```python
from build123d import *

# Parameters (mm, degrees)
SKETCH1_R           = 25
BOSS_EXTRUDE1_DEPTH = 2
SKETCH2_R           = 20
BOSS_EXTRUDE2_DEPTH = 10
SKETCH3_R           = 25
BOSS_EXTRUDE3_DEPTH = 2
SKETCH4_R           = 3.5
CUT_EXTRUDE1_DEPTH  = 19


with BuildPart() as part:
    # Sketch1 → Boss-Extrude1 (new body)
    with BuildSketch(Plane(origin=(0, 0, 0), x_dir=(0, 0, -1), z_dir=(1, 0, 0))):
        Circle(SKETCH1_R)
    extrude(amount=BOSS_EXTRUDE1_DEPTH)

    # Sketch2 → Boss-Extrude2 (add)
    with BuildSketch(Plane(origin=(2, 0, 0), x_dir=(0, 0, -1), z_dir=(1, 0, 0))):
        Circle(SKETCH2_R)
    extrude(amount=BOSS_EXTRUDE2_DEPTH)

    # Sketch3 → Boss-Extrude3 (add)
    with BuildSketch(Plane(origin=(12, 0, 0), x_dir=(0, 0, -1), z_dir=(1, 0, 0))):
        Circle(SKETCH3_R)
    extrude(amount=BOSS_EXTRUDE3_DEPTH)

    # Sketch4 → Cut-Extrude1 (cut)
    with BuildSketch(Plane.ZY):
        Circle(SKETCH4_R)
    extrude(amount=-CUT_EXTRUDE1_DEPTH, mode=Mode.SUBTRACT)


solid = part.part
```
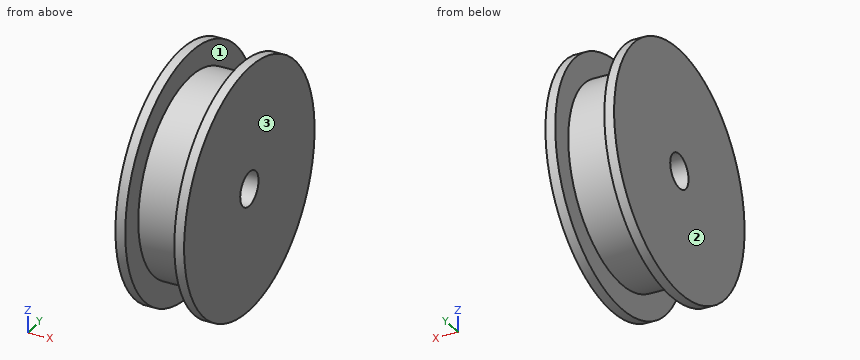
Geometry check sheet. Reference: the model listing, model coordinates, mm. Face numbers are marked on the shaded views. Give positions to 0.01 mm unless a question says otherwise; leave off trailing zeros. Order: outer loops, then holes, each group sorted by start corner. A loop starts at its lowest first (then second) coordinate and runs counter-clockwise, first axis right, second up.
1. Release check for a two-part mould opening along X. For the marked faces 1, 2 and 3 record: pulls with the +X half, pulls with the -X half, needs draft (parallel to the pull), parting line crosses it, or undercut.
2. Section check C-C, the plane x = 4.75. Enter the section's corners in (y, z).
3. Section check A-A, the plane z = 0. Enter the section's corners in (x, y).
4. Thickness scan on L1, parallel to Y at x = 7.75, z = 0; L2, parallel to X at y = 18.5, z = 10.5; L3, parallel to Z at x = 11.5, y = -14. Record the ranges inside material, lowest first.
5. Section check D-D, the plane z = 22.5. Enter the section's corners in (x, y), and give its area (3 significant figures).
6. Gauge pin test, flat ends, axial feed: pin 1 Ø3 at (x, y) = (3, -5.5) entering from -Z; pin 2 Ø6 at (x, y) = (8, -8.5) entering from -Z; pin 3 Ø6.5 at (y, z) = (0, 0) entering from -X; pin 4 Ø1 at (x, y) = (5.5, 12) entering from +Z. Record the tip position at first contact, or that the pin passes through.
Values follow:
1. face 1: undercut
1. face 2: pulls with the -X half
1. face 3: pulls with the +X half
2. outline: circle Ø40 at (0, 0); hole circle Ø7 at (0, 0)
3. outline: (0, -25) - (2, -25) - (2, -20) - (12, -20) - (12, -25) - (14, -25) - (14, -3.5) - (0, -3.5) - close; (0, 3.5) - (14, 3.5) - (14, 25) - (12, 25) - (12, 20) - (2, 20) - (2, 25) - (0, 25) - close
4. L1: y = -20 to -3.5, 3.5 to 20
4. L2: x = 0 to 2, 12 to 14
4. L3: z = -14.28 to 14.28
5. outline: (0, -10.9) - (2, -10.9) - (2, 10.9) - (0, 10.9) - close; (12, -10.9) - (14, -10.9) - (14, 10.9) - (12, 10.9) - close
5. area: 87.2 mm2
6. pin 1: stops at z = -24.61
6. pin 2: stops at z = -19.23
6. pin 3: passes through
6. pin 4: stops at z = 16.36
